Can you work these out from the drawing? Everything is in mm from the part's minimum corner. A direction names the side the tool comes from. Round coordinates to 2 decimals unless told otherwise and drop trailing zeros. Write each loop counter-clockwise with the first axis right and the second up, starting at its lowest first coordinate (ties: lowest second). Pieces come first, ordered by that corner, then holes. Notation, with made-up numbers: M 61.5,76 L 111.5,76 A32 ccw 111.5,112 Z; hole C -0.5,-36.5 d3. An arc over 180 degrees is marked long. Answer in a Markdown table with one row per item. Add a question column.
(1) For the marked faces 4, 5, 6, 7 and 8, which set-ups out of +Z, -Z, +X, -X, +Y, -Y let a thin tool reach every point of the face, with its end or its side?
(2) I'm going to push flat-ended pins straight in: pin 1 (20 mm diameter, centred on x = 12, z = 38.5, fed in from -Y); pin 2 (11 mm diameter, centred on x = 28, y = 22, fed in from +Z); pin 3 (11 mm diameter, centred on x = 24.5, z = 7, fed in from +Y). Where does each tip first touch, or does it pass through?
(3) If I drill on probe 1 along Z at (x, y) = (20, 64.25); probe 2 along Z at (x, y) = (20, 54.5); probe 3 along X at (y, z) = (56, 34), over which ranges is the centre line in solid material (lowest first)?
(4) Suppose I cut it at D-D, the plane z = 34. Write out the boundary of the cut face in (x, y).
(5) If we mould it in two halves opening along Z, with no side actions, what happens to the marked faces 1, 2 and 3? For each: released by +Z, released by -Z, zero draft, split by the parting line, or undercut.
(6) Suppose I cut it at B-B, the plane z = 17. Write out the boundary of the cut face in (x, y).
(7) Suppose I cut it at C-C, the plane y = 59. Write out the boundary of the cut face in (x, z), then the cut area to 3 significant figures.
(8) Suppose I cut it at A-A, the plane x = 20. Write out the boundary of the cut face in (y, z), then the cut area to 3 significant figures.
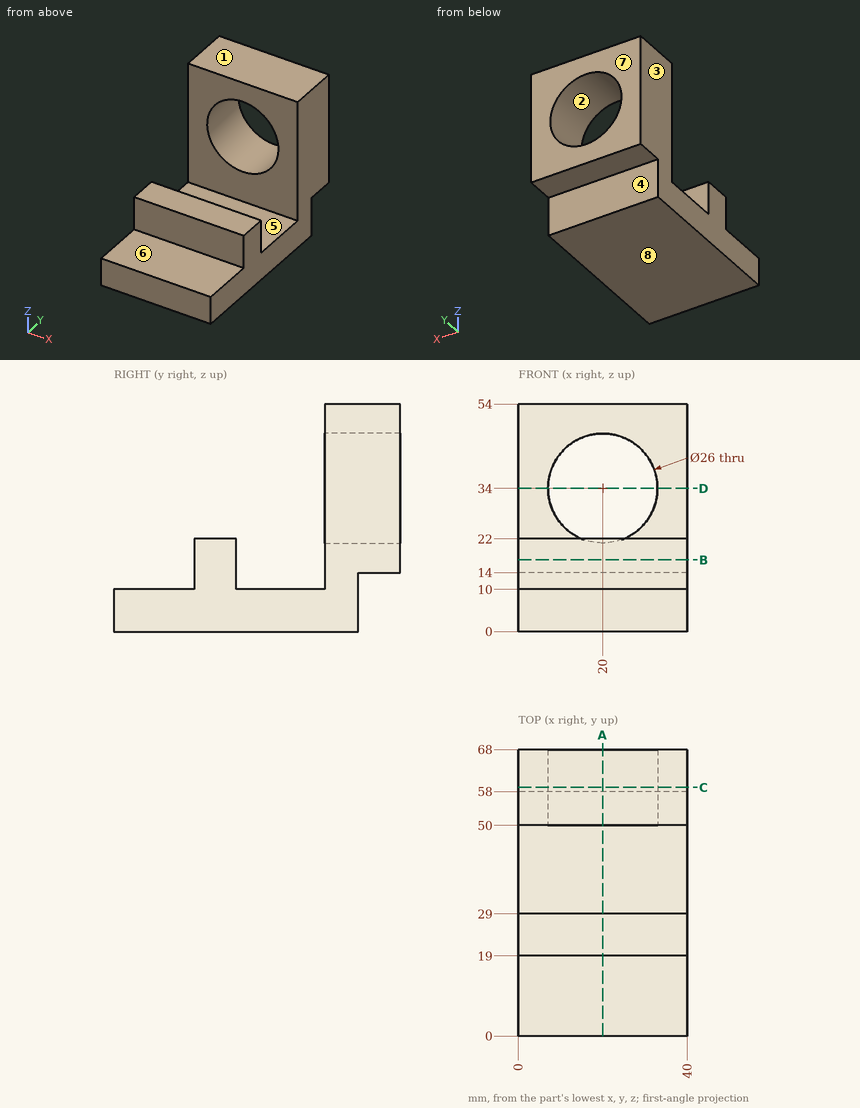
Calculated:
| question | item | result |
|---|---|---|
| 1 | face 4 | -Z, +X, -X, +Y |
| 1 | face 5 | +Z, +X, -X |
| 1 | face 6 | +Z, +X, -X, -Y |
| 1 | face 7 | +Z, -Z, +X, -X, +Y |
| 1 | face 8 | -Z, +X, -X, +Y, -Y |
| 2 | pin 1 | y = 50 |
| 2 | pin 2 | z = 22 |
| 2 | pin 3 | y = 58 |
| 3 | probe 1 | 14 to 21, 47 to 54 |
| 3 | probe 2 | 0 to 21, 47 to 54 |
| 3 | probe 3 | 0 to 7, 33 to 40 |
| 4 | outline | M 0,50 L 7,50 L 7,68 L 0,68 Z; M 33,50 L 40,50 L 40,68 L 33,68 Z |
| 5 | face 1 | released by +Z |
| 5 | face 2 | undercut |
| 5 | face 3 | zero draft |
| 6 | outline | M 0,19 L 40,19 L 40,29 L 0,29 Z; M 0,50 L 40,50 L 40,68 L 0,68 Z |
| 7 | outline | M 0,14 L 40,14 L 40,54 L 0,54 Z; hole C 20,34 d26 |
| 7 | area | 1,070 mm² |
| 8 | outline | M 0,0 L 58,0 L 58,14 L 68,14 L 68,21 L 50,21 L 50,10 L 29,10 L 29,22 L 19,22 L 19,10 L 0,10 Z; M 50,47 L 68,47 L 68,54 L 50,54 Z |
| 8 | area | 984 mm² |
